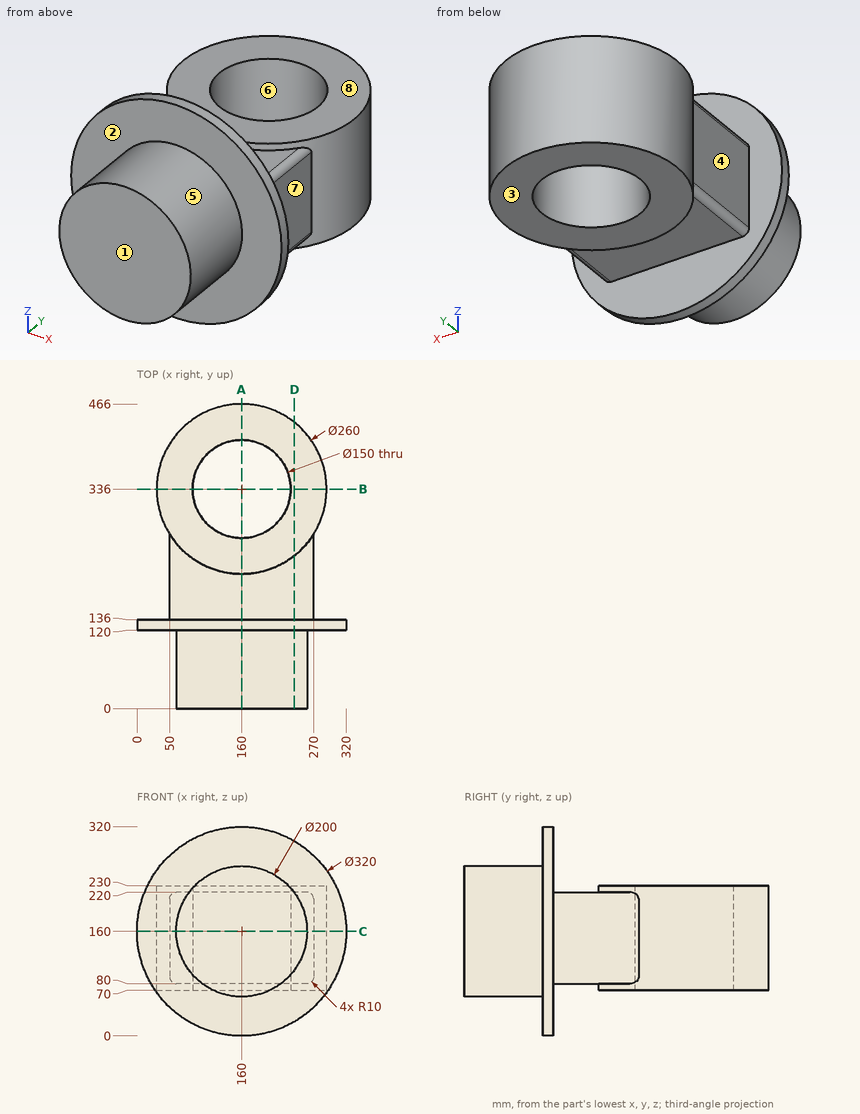
Job drawing, mm, ordinate dimensions from the low corner. One solid piece. A direction names the side the tool comes from. Give positions to 0.01 mm unless a question says otherwise; leave off trailing zeros. Loops run counter-clockwise (first coordinate to the right, second up) from the corner with the lowest first, then second, coordinate; pieces in that order, holes last. Notation, with made-up numbers: (23.5, -40) -> (80.5, -40) arc R35 cw to (80.5, -3) -> close; hole circle Ø10 at (34.25, 42). An arc over 180 degrees is marked (long way). Write each question's results on one line, items separated by ' | '. Start each with the question number.
Q1. Which spindle directions (+Z, -Z, +X, -X, +Y, -Y) get a long thin tool onto all of the face, cutting with end or side? Do the marked faces 1, 2, 3 and 4. Say none if no direction does.
Q2. Wall check: L1, parallel to X at y = 336, z = 121; L2, parallel to Y at x = 160, z = 184; L3, parallel to X at y = 326, z = 74. Give the ranges that are in metal, low to high.
Q3. Pull direction X, two halves, no side cores. Call the marked faces 5, 6, 7 and 8: +X half, -X half, draft (parallel to the pull), parting line (faces both ways), or undercut.
Q4. Pin check, flat tips, straight feed: P1, Ø12, axis at x = 168.5, y = 101.5, coming from the +Z side; P2, Ø5, axis at x = 236, y = 359.5, coming from the -Z side; P3, Ø2, axis at x = 144.5, z = 139, coming from the -Y side; P4, Ø4, axis at x = 263.5, z = 186.5, coming from the +Y side. Stop position of each tip, or through.
Q5. Band-saw the part on B-B on y = 336. List the corners of the cut face in (x, z), plus the area to 3 significant figures.
Q6. Band-saw the part on D-D on x = 240.5. List the corners of the cut face in (y, z), plus the area to 3 significant figures.
Q7. Band-saw the part on C-C on z = 160. List the corners of the cut face in (x, y), plus the area to 3 significant figures.
Q8. Band-saw the part on A-A on x = 160. List the corners of the cut face in (y, z).
Results are:
1) face 1: +Z, -Z, +X, -X, -Y | face 2: -Y | face 3: -Z, +X, -X, +Y | face 4: +Z, -Z, -X
2) L1: x = 30 to 85, 235 to 290 | L2: y = 0 to 261, 411 to 466 | L3: x = 30.39 to 85.67, 234.33 to 289.61
3) face 5: parting line | face 6: undercut | face 7: +X half | face 8: draft
4) P1: stops at z = 259.97 | P2: stops at z = 70 | P3: stops at y = 0 | P4: stops at y = 417.23
5) outline: (30, 70) -> (85, 70) -> (85, 230) -> (30, 230) -> close; (235, 70) -> (290, 70) -> (290, 230) -> (235, 230) -> close | area: 17,600 mm²
6) outline: (0, 100.67) -> (120, 100.67) -> (120, 21.73) -> (136, 21.73) -> (136, 80) -> (233.92, 80) -> (233.92, 70) -> (438.08, 70) -> (438.08, 230) -> (233.92, 230) -> (233.92, 220) -> (136, 220) -> (136, 298.27) -> (120, 298.27) -> (120, 219.33) -> (0, 219.33) -> close | area: 65,000 mm²
7) outline: (0, 120) -> (60, 120) -> (60, 0) -> (260, 0) -> (260, 120) -> (320, 120) -> (320, 136) -> (270, 136) -> (270, 266.72) arc R130 ccw (long way) to (50, 266.72) -> (50, 136) -> (0, 136) -> close; hole circle Ø150 at (160, 336) | area: 83,900 mm²
8) outline: (0, 60) -> (120, 60) -> (120, 0) -> (136, 0) -> (136, 80) -> (206, 80) -> (206, 70) -> (261, 70) -> (261, 230) -> (206, 230) -> (206, 220) -> (136, 220) -> (136, 320) -> (120, 320) -> (120, 260) -> (0, 260) -> close; (411, 70) -> (466, 70) -> (466, 230) -> (411, 230) -> close
